from build123d import *

# Parameters (mm, degrees)
F0_W     = 20
F0_H     = 3
F0_W_2   = 12
F0_W_3   = 15
F0_H_2   = 5
F1_DEPTH = 3


with BuildPart() as f1:
    # F0 (on Front) → F1 (new body)
    with BuildSketch(Plane.XZ):
        with BuildLine():
            ThreePointArc((76.362, 36.409888), (73.433068, 43.480956), (66.362, 46.409888))
            Line((66.362, 46.409888), (-63.638, 46.409888))
            ThreePointArc((-63.638, 46.409888), (-70.709067, 43.480956), (-73.638, 36.409888))
            Line((-73.638, 36.409888), (-73.638, -43.590112))
            ThreePointArc((-73.638, -43.590112), (-70.709067, -50.66118), (-63.638, -53.590112))
            Line((-63.638, -53.590112), (66.362, -53.590112))
            ThreePointArc((66.362, -53.590112), (73.433068, -50.66118), (76.362, -43.590112))
            Line((76.362, -43.590112), (76.362, 36.409888))
        make_face()
        with Locations((-45.638, -36.090112)):
            Rectangle(F0_W, F0_H, mode=Mode.SUBTRACT)
        with Locations((-61.638, -24.590112)):
            Rectangle(F0_W_2, F0_H, mode=Mode.SUBTRACT)
        with Locations((36.362, -35.090112)):
            Rectangle(F0_W_3, F0_H_2, mode=Mode.SUBTRACT)
        with Locations((-61.638, 17.409888)):
            Rectangle(F0_W_2, F0_H, mode=Mode.SUBTRACT)
        with Locations((-45.638, 28.909888)):
            Rectangle(F0_W, F0_H, mode=Mode.SUBTRACT)
        with Locations((36.362, 27.909888)):
            Rectangle(F0_W_3, F0_H_2, mode=Mode.SUBTRACT)
    extrude(amount=F1_DEPTH)


solid = f1.part
CAD build for the part. Positions are in the model's coordinates, mm. A direction names the side the tool comes from. Give positions to 0.01 mm unless a question says otherwise; leave off trailing zeros. Write each loop counter-clockwise with the first axis right and the second up, starting at its lowest first coordinate (ties: lowest second). Pieces come first, ordered by that corner, then holes. Notation, with made-up numbers: (43.25, -5) -> (68.25, -5) arc R16 ccw to (68.25, 2) -> close; hole circle Ø5 at (32, 64). An arc over 180 degrees is marked (long way). Return JSON: item names as keys, results as strings.
Item 1: Band-saw the part on B-B (y = -1.65). Give the number of separate pieces and of enclosed holes in the cut face, then the cut area to 3 significant figures.
Answer below:
{"separate pieces": "1", "enclosed holes": "6", "area": "14,600 mm2"}
Item 2: Two-plate mould, pull along X, no slides. Class faces 1 (the flat face through (0, 0, -3)), 2 (the flat face through (36, -1, -37.59)), 3 (the flat face through (28.862, -1, -35)), 4 (the cylindrical face through (73.51, -1.479, 43.403)): +X half, -X half, draft (parallel to the pull), parting line (faces both ways), or undercut.
Answer below:
{"face 1": "draft", "face 2": "undercut", "face 3": "undercut", "face 4": "+X half"}
Item 3: Tool access for faces 5 (the flat face through (-73.638, -1, -3)), 6 (the flat face through (-62, -1, -23.09)): list every direction of +Z, -Z, +X, -X, +Y, -Y with a clear straight run to the whole face (end or side of a thin tool).
Answer below:
{"face 5": "+Z, -Z, -X, +Y, -Y", "face 6": "+Y, -Y"}
Item 4: Band-saw the part on C-C (x = 40.5). List the corners of the cut face in (y, z).
Answer below:
{"outline": "(-3, -53.59) -> (0, -53.59) -> (0, -37.59) -> (-3, -37.59) -> close; (-3, -32.59) -> (0, -32.59) -> (0, 25.41) -> (-3, 25.41) -> close; (-3, 30.41) -> (0, 30.41) -> (0, 46.41) -> (-3, 46.41) -> close"}
Item 5: Band-saw the part on A-A (x = -37.5). List the corners of the cut face in (y, z), then the cut area to 3 significant figures.
Answer below:
{"outline": "(-3, -53.59) -> (0, -53.59) -> (0, -37.59) -> (-3, -37.59) -> close; (-3, -34.59) -> (0, -34.59) -> (0, 27.41) -> (-3, 27.41) -> close; (-3, 30.41) -> (0, 30.41) -> (0, 46.41) -> (-3, 46.41) -> close", "area": "282 mm2"}
Item 6: Drill centre lines: probe 1 along Z at (x, y) = (36, -0.25); probe 2 along Z at (x, y) = (-54, -2.05); probe 3 along X at (y, z) = (-1.8, 36.5). Where is each one in solid material? Low to high.
Answer below:
{"probe 1": "z = -53.59 to -37.59, -32.59 to 25.41, 30.41 to 46.41", "probe 2": "z = -53.59 to -37.59, -34.59 to 27.41, 30.41 to 46.41", "probe 3": "x = -73.64 to 76.36"}
